Build history of the part. All positions in model axes, mm. A direction names the side the tool comes from. Give positions to 0.01 mm unless a question says otherwise; leave off trailing zeros. Order: outer loops, then holes, each group sorted by start corner. A loop starts at its lowest first (then second) coordinate and runs counter-clockwise, first axis right, second up. Notation, with made-up numbers: (5, -15.5) - (42, -15.5) arc R21 ccw to (42, 22.5) - close; hole circle Ø3 at (-27.75, -16.5). An arc over 180 degrees is marked (long way). Answer in a Markdown table with one row per item.
```python
from build123d import *

# Parameters (mm, degrees)
F0_W     = 66.3122907281
F0_H     = 100.8766070008
F0_R     = 5.5402980892
F1_DEPTH = 64.77
F3_DEPTH = 75.692
F5_DEPTH = 65.786
F7_DEPTH = 101.6


with BuildPart() as f1:
    # F0 (on Top) → F1 (new body)
    with BuildSketch(Plane.XY):
        Rectangle(F0_W, F0_H)
        with Locations((0, -39.684958756)):
            Circle(F0_R, mode=Mode.SUBTRACT)
        with Locations((0, 39.684958756)):
            Circle(F0_R, mode=Mode.SUBTRACT)
    extrude(amount=F1_DEPTH)

    # F2 (on face) → F3 (join, symmetric)
    with BuildSketch(Plane.YZ.offset(33.156145364)):
        with BuildLine():
            Line((8.4750251617, 64.77), (-8.4750251617, 64.77))
            ThreePointArc((-8.4750251617, 64.77), (0, 56.2949748383), (8.4750251617, 64.77))
        make_face()
        with BuildLine():
            ThreePointArc((8.4750251617, 64.77), (0, 56.2949748383), (-8.4750251617, 64.77))
            Line((-8.4750251617, 64.77), (-14.2677179965, 64.77))
            ThreePointArc((-14.2677179965, 64.77), (0, 50.5022820035), (14.2677179965, 64.77))
            Line((14.2677179965, 64.77), (8.4750251617, 64.77))
        make_face()
    extrude(amount=F3_DEPTH, both=True)

    # F4 (on face) → F5 (cut)
    with BuildSketch(Plane.YZ.offset(108.848145364)):
        with BuildLine():
            Line((14.2677179965, 64.77), (-14.2677179965, 64.77))
            ThreePointArc((-14.2677179965, 64.77), (0, 50.5022820035), (14.2677179965, 64.77))
        make_face()
    extrude(amount=-F5_DEPTH, mode=Mode.SUBTRACT)

    # F6 (on face) → F7 (cut)
    with BuildSketch(Plane.YZ.offset(43.062145364)):
        with BuildLine():
            Line((8.7146712467, 64.77), (-8.7146712467, 64.77))
            ThreePointArc((-8.7146712467, 64.77), (0, 56.0553287533), (8.7146712467, 64.77))
        make_face()
    extrude(amount=-F7_DEPTH, mode=Mode.SUBTRACT)


solid = f1.part
```
1. Cut at C-C on z = 30. Write the cut outline in (x, y), and give its area (3 significant figures).
Check result:
| item | result |
|---|---|
| outline | (-33.16, -50.44) - (33.16, -50.44) - (33.16, 50.44) - (-33.16, 50.44) - close; hole circle Ø11.08 at (0, -39.68); hole circle Ø11.08 at (0, 39.68) |
| area | 6,500 mm² |
2. Drop flat-ended pins along their axis: P1, Ø1, axis at y = 32.5, z = 19.5, coming from the -X side; P2, Ø10, axis at x = -33, y = -2, coming from the +Z side; P3, Ø3, axis at x = 19, y = -3.5, coming from the +Z side; P4, Ø10, axis at x = 0, y = 39.68, coming from the -Z side. Give the stop position or say it passes through.
Check result:
| item | result |
|---|---|
| P1 | stops at x = -33.16 |
| P2 | stops at z = 59.58 |
| P3 | stops at z = 57.63 |
| P4 | passes through |
3. Which spindle directions (+Z, -Z, +X, -X, +Y, -Y) get a long thin tool onto all of the face, cutting with end or side? Do faces 1 (the face through (43.062, 0, 55)), 2 (the face through (-37.78, -0.314, 50.506)). Say none if no direction does.
Check result:
| item | result |
|---|---|
| face 1 | +Z, -Z, +X, +Y, -Y |
| face 2 | -Z, -X |
4. Cut at B-B on y = 0. Write the cut outline in (x, z), and give its area (3 significant figures).
Check result:
| item | result |
|---|---|
| outline | (-42.54, 50.5) - (-33.16, 50.5) - (-33.16, 0) - (33.16, 0) - (33.16, 50.5) - (43.06, 50.5) - (43.06, 56.06) - (-42.54, 56.06) - close |
| area | 3,820 mm² |
5. Probe line 1 (Y direction, x = 0, z = 30.5); line 2 (Y direction, x = 4.5, z = 50); line 3 (X direction, y = 12, z = 10). List the from-to ranges inside material, lowest first.
Check result:
| item | result |
|---|---|
| line 1 | y = -50.44 to -45.23, -34.14 to 34.14, 45.23 to 50.44 |
| line 2 | y = -50.44 to -42.92, -36.45 to 36.45, 42.92 to 50.44 |
| line 3 | x = -33.16 to 33.16 |
6. Cut at D-D on z = 54.5. Write the cut outline in (x, y), and give its area (3 significant figures).
Check result:
| item | result |
|---|---|
| outline | (-42.54, -9.9) - (-33.16, -9.9) - (-33.16, -50.44) - (33.16, -50.44) - (33.16, -9.9) - (43.06, -9.9) - (43.06, 9.9) - (33.16, 9.9) - (33.16, 50.44) - (-33.16, 50.44) - (-33.16, 9.9) - (-42.54, 9.9) - close; hole circle Ø11.08 at (0, -39.68); hole circle Ø11.08 at (0, 39.68) |
| area | 6,880 mm² |
7. Two-plate mould, pull along Y, no slides. Class faces 3 (the face through (-1.201, -45.094, 31.932)), 4 (the face through (38.178, -0.314, 50.506)), 5 (the face through (1, -29, 64.77)): +Y half, -Y half, draft (parallel to the pull), parting line (faces both ways), or undercut.
Check result:
| item | result |
|---|---|
| face 3 | undercut |
| face 4 | parting line |
| face 5 | draft |
8. Cut at A-A on x = 0. Write the cut outline in (y, z).
Check result:
| item | result |
|---|---|
| outline | (-50.44, 0) - (-45.23, 0) - (-45.23, 64.77) - (-50.44, 64.77) - close; (-34.14, 0) - (34.14, 0) - (34.14, 64.77) - (8.71, 64.77) arc R8.71 cw to (-8.71, 64.77) - (-34.14, 64.77) - close; (45.23, 0) - (50.44, 0) - (50.44, 64.77) - (45.23, 64.77) - close |
